The model under review builds one solid part; all positions refer to its coordinate system, in mm. A direction names the side the tool comes from. Coordinates: 2 decimals unless noted, no trailing zeros. Loops run counter-clockwise (first coordinate to the right, second up) from the corner with the lowest first, then second, coordinate; pieces in that order, holes last. Notation, with made-up numbers: M 53,-37 L 86,-37 A31 ccw 86,-9 Z; hole C 80,13.5 d4. An arc over 180 degrees is marked long. Return JSON: item names as keys, results as strings.
```python
from build123d import *

# Parameters (mm, degrees)
BOSS_EXTRUDE1_DEPTH = 304.8
SKETCH2_R           = 4
CUT_EXTRUDE1_DEPTH  = 308.50494305
SKETCH3_R           = 4
CUT_EXTRUDE2_DEPTH  = 308.50494305


with BuildPart() as part:
    # Sketch1 → Boss-Extrude1 (new body)
    with BuildSketch(Plane.XY):
        Polygon((0, 0), (0, 30), (2.5, 30), (2.5, 2.5), (30, 2.5), (30, 0), align=None)
    extrude(amount=BOSS_EXTRUDE1_DEPTH)

    # Sketch2 → Cut-Extrude1 (cut, through all)
    with BuildSketch(Plane(origin=(0, 2.5, 0), x_dir=(1, 0, 0), z_dir=(0, 1, 0))):
        with Locations(Location((20, -17.5, 0), (0, 0, 180))):
            Circle(SKETCH2_R)
    extrude(amount=-CUT_EXTRUDE1_DEPTH, mode=Mode.SUBTRACT)

    # Sketch3 → Cut-Extrude2 (cut, through all)
    with BuildSketch(Plane(origin=(2.5, 0, 0), x_dir=(0, 0, -1), z_dir=(1, 0, 0))):
        with Locations(Location((-12.5, 17.5, 0), (0, 0, 90))):
            Circle(SKETCH3_R)
    extrude(amount=-CUT_EXTRUDE2_DEPTH, mode=Mode.SUBTRACT)


solid = part.part
```
1. The part is to be moulded in two halves that separate along Z. For faces 3 (the face through (8, 2, 304.8)), 4 (the face through (1.27, 14.55, 15.2)), 5 (the face through (8, 2, 0)), say which applies: released by +Z, released by -Z, zero draft, split by the parting line, or undercut.
Check values:
{"face 3": "released by +Z", "face 4": "undercut", "face 5": "released by -Z"}
2. Add section B-B on x = 20. Give the boundary of the cut face in (y, z), plus the area to 3 significant figures.
Check values:
{"outline": "M 0,0 L 2.5,0 L 2.5,13.5 L 0,13.5 Z; M 0,21.5 L 2.5,21.5 L 2.5,304.8 L 0,304.8 Z", "area": "742 mm²"}
3. Machinability: for faces 1 (the face through (2.5, 16, 150)), 2 (the face through (0, 15, 150)), which of the approach directions +Z, -Z, +X, -X, +Y, -Y give a long, thin tool a straight path to every point of the face, cutting with its end or side? Answer none if there is none.
Check values:
{"face 1": "+Z, -Z, +X, +Y", "face 2": "+Z, -Z, -X, +Y, -Y"}
4. Add section D-D on y = 6. Give the boundary of the cut face in (x, z), plus the area to 3 significant figures.
Check values:
{"outline": "M 0,0 L 2.5,0 L 2.5,304.8 L 0,304.8 Z", "area": "762 mm²"}
5. Add section A-A on y = 17.5. Give the boundary of the cut face in (x, z), plus the area to 3 significant figures.
Check values:
{"outline": "M 0,0 L 2.5,0 L 2.5,8.5 L 0,8.5 Z; M 0,16.5 L 2.5,16.5 L 2.5,304.8 L 0,304.8 Z", "area": "742 mm²"}
6. Add section C-C on z = 243. Give the boundary of the cut face in (x, y).
Check values:
{"outline": "M 0,0 L 30,0 L 30,2.5 L 2.5,2.5 L 2.5,30 L 0,30 Z"}
7. To check wall thickness, follow line 1 (Z direction, x = 1.3, y = 17.5); line 2 (Z direction, x = 20, y = 1); line 3 (Y direction, x = 21.25, z = 254.5). State the ranges of each line that lie inside material, in increasing order.
Check values:
{"line 1": "0 to 8.5, 16.5 to 304.8", "line 2": "0 to 13.5, 21.5 to 304.8", "line 3": "0 to 2.5"}
8. Insertion check: pin 1 Ø6 at (x, z) = (17.5, 267.5) entering from +Y; pin 2 Ø6.5 at (y, z) = (17.5, 12.5) entering from -X; pin 3 Ø8 at (y, z) = (10.5, 103.5) entering from +X. Each pin has a flat end and moves straight along its axis. Give the tip position at first contact, or say it passes through.
Check values:
{"pin 1": "y = 2.5", "pin 2": "through", "pin 3": "x = 2.5"}
